```python
from build123d import *

# Parameters (mm, degrees)
SKETCH_W        = 107
SKETCH_H        = 95
PAD_DEPTH       = 7
THICKNESS_T     = 3.5
SKETCH001_R     = 6.56
POCKET_DEPTH    = 5
SKETCH002_W     = 12.979027
SKETCH002_H     = 7.757147
POCKET001_DEPTH = 5


with BuildPart() as part:
    # Sketch → Pad (new body, symmetric)
    with BuildSketch(Plane.XY):
        with Locations((146.021704, -118.608821)):
            Rectangle(SKETCH_W, SKETCH_H)
    extrude(amount=PAD_DEPTH, both=True)

    # Thickness
    thickness_openings = [part.faces().sort_by_distance(p)[0] for p in [
        (146.021704, -118.608821, -7),
    ]]
    offset(amount=THICKNESS_T, openings=thickness_openings)

    # Sketch001 (on Face18 of Thickness) → Pocket (cut)
    with BuildSketch(Plane.XY.offset(10.5)):
        with Locations((145.68, -152.08)):
            Circle(SKETCH001_R)
        Polygon((95.8, -101.98), (195.32, -101.98), (195.32, -142.15), (186.15, -142.15), (186.15, -162.39), (163.22, -162.39), (163.22, -142.15), (127.9, -142.15), (127.9, -162.39), (104.97, -162.39), (104.97, -142.15), (95.8, -142.15), align=None)
    extrude(amount=-POCKET_DEPTH, mode=Mode.SUBTRACT)

    # Sketch002 (on Face11 of Pocket) → Pocket001 (cut)
    with BuildSketch(Plane(origin=(89.021704, 0, 0), x_dir=(0, -1, 0), z_dir=(-1, 0, 0))):
        with Locations((90.140796, 3.473584)):
            Rectangle(SKETCH002_W, SKETCH002_H)
    extrude(amount=-POCKET001_DEPTH, mode=Mode.SUBTRACT)


solid = part.part
```
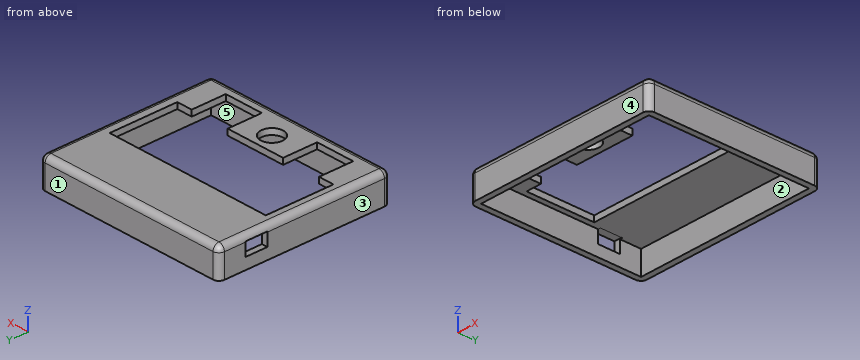
Here's how the part is built. I have some questions about the finished solid (model axes, mm). Face numbers are marked on the shaded views. A direction names the side the tool comes from. Give positions to 0.01 mm unless a question says otherwise; leave off trailing zeros. Write each loop counter-clockwise with the first axis right and the second up, starting at its lowest first coordinate (ties: lowest second). Pieces come first, ordered by that corner, then holes. Notation, with made-up numbers: M -22.5,3 L -10.5,3 A16 ccw -10.5,18 Z; hole C 17.25,43.5 d11. An arc over 180 degrees is marked long. Put each result on its own line as item: value. Start each with the question number.
Item 1: If we section it at D-D, the plane y = -122: Write out the boundary of the cut face in (x, z).
Item 2: If we section it at B-B, the plane z = -5.5: Write out the boundary of the cut face in (x, y).
Item 3: On a 3-axis mill with a long thin cutter (end or side, diameter ignored), from which of +Z, -Z, +X, -X, +Y, -Y can I reach the whole of each face in a straight line? I mean the marked faces 1 and 2. Say none if no direction works.
Item 4: If we section it at A-A, the plane y = -152.08: Write out the boundary of the cut face in (x, z).
Item 5: I need wall thicknesses on L1, parallel to Y at x = 167.5, z = -2; L2, parallel to X at y = -152.5, z = 9.25; L3, parallel to Y at x = 145.68, z = 9.4. Which ranges of each line are inside material? Lowest first, please. Write a range as from..to.
Item 6: Will these pins go through, and if not, where does the flat tip stop? pin 1 (1 mm diameter, centred on x = 137.5, z = 8.5, fed in from -Y); pin 2 (1 mm diameter, centred on y = -121, z = 9, fed in from -X); pin 3 (1.8 mm diameter, centred on x = 121, z = 9.5, fed in from +Y).
Item 7: Thinking about a two-plate mould opening in X: for the marked faces 3, 4 and 5, which applies, +X half, -X half, draft (parallel to the pull), parting line (faces both ways), or undercut?
Item 8: If we section it at C-C, the plane x = 145.68: Write out the boundary of the cut face in (y, z), then the cut area to 3 significant figures.
Values:
1. outline: M 89.02,-7 L 92.52,-7 L 92.52,7 L 95.8,7 L 95.8,10.5 L 92.52,10.5 A3.5 ccw 89.02,7 Z; M 195.32,7 L 199.52,7 L 199.52,-7 L 203.02,-7 L 203.02,7 A3.5 ccw 199.52,10.5 L 195.32,10.5 Z
2. outline: M 89.02,-166.11 A3.5 ccw 92.52,-169.61 L 199.52,-169.61 A3.5 ccw 203.02,-166.11 L 203.02,-71.11 A3.5 ccw 199.52,-67.61 L 92.52,-67.61 A3.5 ccw 89.02,-71.11 Z; hole M 92.52,-166.11 L 199.52,-166.11 L 199.52,-71.11 L 92.52,-71.11 Z
3. face 1: +Z, -Z, +X, -X, +Y
3. face 2: -Z
4. outline: M 89.02,-7 L 92.52,-7 L 92.52,7 L 104.97,7 L 104.97,10.5 L 92.52,10.5 A3.5 ccw 89.02,7 Z; M 127.9,7 L 139.12,7 L 139.12,10.5 L 127.9,10.5 Z; M 152.24,7 L 163.22,7 L 163.22,10.5 L 152.24,10.5 Z; M 186.15,7 L 199.52,7 L 199.52,-7 L 203.02,-7 L 203.02,7 A3.5 ccw 199.52,10.5 L 186.15,10.5 Z
5. L1: -169.61..-166.11, -71.11..-67.61
5. L2: 89.84..104.97, 127.9..139.13, 152.23..163.22, 186.15..202.2
5. L3: -168.66..-158.64, -145.52..-142.15, -101.98..-68.56
6. pin 1: y = -169.46
6. pin 2: x = 89.36
6. pin 3: y = -68
7. face 3: -X half
7. face 4: draft
7. face 5: undercut
8. outline: M -169.61,-7 L -166.11,-7 L -166.11,7 L -158.64,7 L -158.64,10.5 L -166.11,10.5 A3.5 ccw -169.61,7 Z; M -145.52,7 L -142.15,7 L -142.15,10.5 L -145.52,10.5 Z; M -101.98,7 L -71.11,7 L -71.11,-7 L -67.61,-7 L -67.61,7 A3.5 ccw -71.11,10.5 L -101.98,10.5 Z
8. area: 263 mm²
